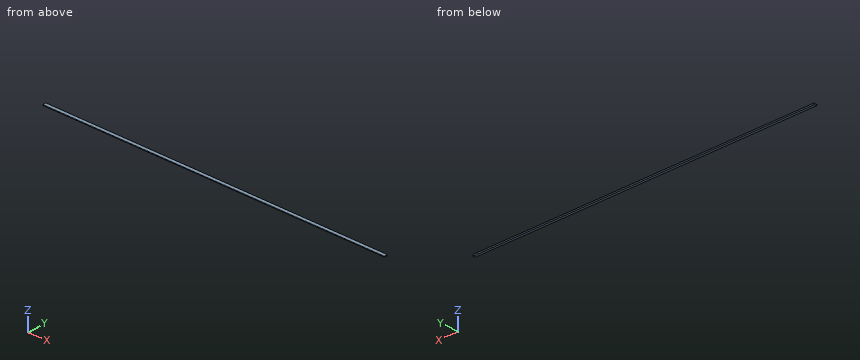
```python
from build123d import *

# Parameters (mm, degrees)
F1_DEPTH = 1203.325


with BuildPart() as f1:
    # F0 (on Right) → F1 (new body, symmetric)
    with BuildSketch(Plane.YZ):
        with BuildLine():
            ThreePointArc((-16.66875, 0), (-17.6251806772, 2.097476653), (-19.8359280858, 2.7507483004))
            ThreePointArc((-19.8359280858, 2.7507483004), (-22.225, 0), (-19.8359280858, -2.7507483004))
            ThreePointArc((-19.8359280858, -2.7507483004), (-17.6251806772, -2.097476653), (-16.66875, 0))
        make_face()
        with BuildLine():
            Line((-0.8483794827, -5.4362591395), (0, 0))
            Line((0, 0), (-0.8483794827, 5.4362591395))
            Line((-0.8483794827, 5.4362591395), (-19.8359280858, 2.7507483004))
            ThreePointArc((-19.8359280858, 2.7507483004), (-17.6251806772, 2.097476653), (-16.66875, 0))
            ThreePointArc((-16.66875, 0), (-17.6251806772, -2.097476653), (-19.8359280858, -2.7507483004))
            Line((-19.8359280858, -2.7507483004), (-0.8483794827, -5.4362591395))
        make_face()
    extrude(amount=F1_DEPTH, both=True)


solid = f1.part
```
Geometry check sheet. Reference: the model listing, model coordinates, mm. Coordinates: 2 decimals unless noted, no trailing zeros. Order: outer loops, then holes, each group sorted by start corner. A loop starts at its lowest first (then second) coordinate and runs counter-clockwise, first axis right, second up. Notation, with made-up numbers: (63.5, 18) - (110.5, 18) arc R19 cw to (110.5, 29) - close; hole circle Ø3 at (46.25, 20.5). An arc over 180 degrees is marked (long way). Answer in a Markdown table with one row per item. Add a question column.
1. Material ranges on L1, parallel to Y at x = 733, z = 0.75; L2, parallel to Y at x = 607.5, z = 1.5; L3, parallel to Z at x = -519.5, y = -16.5, recorded low to high. Write a range as [from, to].
2. Section check B-B (y = -15.5). Enter the section's corners in (x, z) (3 decimals), plus the area to 3 significant figures.
3. Section check A-A (x = -787). Enter the section's corners in (y, z).
4. Gauge pin test, flat ends, axial feed: pin 1 Ø1 at (x, y) = (413, -20) entering from +Z; pin 2 Ø12 at (x, y) = (-304.5, -14) entering from +Z; pin 3 Ø12 at (x, y) = (-621.5, -17.5) entering from -Z; pin 4 Ø1 at (x, z) = (227.5, 0.5) entering from -Y (3 decimals). Record the tip position at first contact, or that the pin passes through.
Data:
| question | item | result |
|---|---|---|
| 1 | L1 | y = [-22.12, -0.12] |
| 1 | L2 | y = [-21.79, -0.23] |
| 1 | L3 | z = [-3.22, 3.22] |
| 2 | outline | (-1203.325, -3.364) - (1203.325, -3.364) - (1203.325, 3.364) - (-1203.325, 3.364) - close |
| 2 | area | 16,200 mm² |
| 3 | outline | (-19.84, -2.75) - (-0.85, -5.44) - (0, 0) - (-0.85, 5.44) - (-19.84, 2.75) arc R2.78 ccw to start |
| 4 | pin 1 | stops at z = 2.8 |
| 4 | pin 2 | stops at z = 4.42 |
| 4 | pin 3 | stops at z = -3.93 |
| 4 | pin 4 | stops at y = -22.225 |
